from build123d import *

# Parameters (mm, degrees)
F0_W     = 90
F0_H     = 60
F1_DEPTH = 10
F2_R     = 1
F3_DEPTH = 4


with BuildPart() as f1:
    # F0 (on Top) → F1 (new body)
    with BuildSketch(Plane.XY):
        Rectangle(F0_W, F0_H)
    extrude(amount=F1_DEPTH)

    # F2 (on face) → F3 (join)
    with BuildSketch(Plane.XY.offset(10)):
        with Locations((-14, 0)):
            Circle(F2_R)
        with Locations((14, 0)):
            Circle(F2_R)
        with Locations((-32, 0)):
            Circle(F2_R)
        with Locations((32, 0)):
            Circle(F2_R)
    extrude(amount=F3_DEPTH)


solid = f1.part
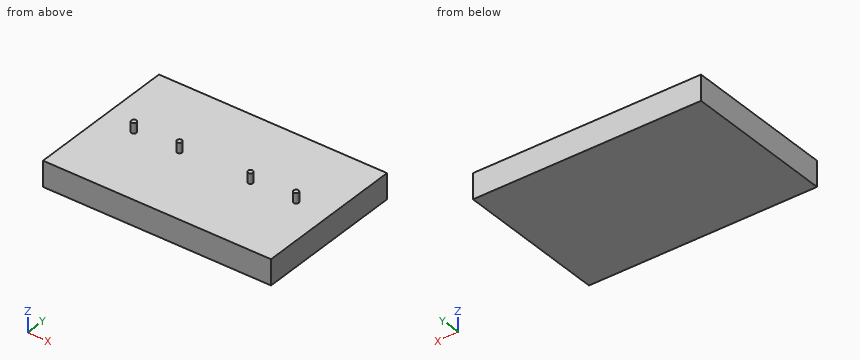
Verification items for the finished model (mm, model axes). Give positions to 0.01 mm unless a question says otherwise; leave off trailing zeros. Write each loop counter-clockwise with the first axis right and the second up, starting at its lowest first coordinate (ties: lowest second). Pieces come first, ordered by that corner, then holes. Notation, with made-up numbers: M 63.25,16 L 109.25,16 A17 cw 109.25,47 Z; hole C -4,70 d6. An arc over 180 degrees is marked long. Use CSV: the item, a comma, the result in double quotes.
1) Cross-section at A-A (x = -14). Enter the section's corners in (y, z), plus the area to 3 significant figures.
Final values:
outline,"M -30,0 L 30,0 L 30,10 L 1,10 L 1,14 L -1,14 L -1,10 L -30,10 Z"
area,"608 mm²"
2) Cross-section at B-B (y = 0). Enter the section's corners in (x, z), plus the area to 3 significant figures.
Final values:
outline,"M -45,0 L 45,0 L 45,10 L 33,10 L 33,14 L 31,14 L 31,10 L 15,10 L 15,14 L 13,14 L 13,10 L -13,10 L -13,14 L -15,14 L -15,10 L -31,10 L -31,14 L -33,14 L -33,10 L -45,10 Z"
area,"932 mm²"
3) Material ranges on line 1 along Z through (x, y) = (39, -5), recorded low to high.
Final values:
line 1,"0 to 10"
4) Cross-section at C-C (y = 23.5). Enter the section's corners in (x, z), plus the area to 3 significant figures.
Final values:
outline,"M -45,0 L 45,0 L 45,10 L -45,10 Z"
area,"900 mm²"
